Input: part model. Units: mm. Frame: model coordinates. A direction names the side the tool comes from. Round coordinates to 2 decimals unless told otherwise and drop trailing zeros. Loops run counter-clockwise (first coordinate to the right, second up) from the corner with the lowest first, then second, coordinate; pieces in that order, holes last. Notation, with made-up numbers: (59.25, 42) -> (78.25, 42) arc R17 ccw to (78.25, 67) -> close; hole circle Ø9 at (-30.5, -14). An arc over 180 degrees is marked (long way). Answer as a JSON object with one key per item and string values. Group by question number.
Item 1: Draft query along Y for faces 5 (the flat face through (-8, 27, 3.175)), 6 (the cylindrical face through (-51.7, 122.3, 0)), 7 (the cylindrical face through (45.26, 111.96, 0.83)), 8 (the cylindrical face through (40.365, 31.913, 0.827)). Return one class per face: released by +Y, released by -Y, zero draft, split by the parting line, or undercut.
Item 2: Section query C-C on y = 71. Return loops of the section in (x, z) (3 decimals).
Item 3: Pin query (flat end, axial travel): pin 1 (6 mm diameter, centred on x = 42.52, y = 30.54, fed in from +Z) (3 decimals); pin 2 (8 mm diameter, centred on x = -96.27, y = 37.1, fed in from -Z); pin 3 (4 mm diameter, centred on x = 46.02, y = 109.52, fed in from +Z); pin 4 (2 mm diameter, centred on x = 34, z = 0, fed in from +Y). Return the tip coordinate at first contact, or that it passes through.
Item 4: Section query A-A on x = 25.5. Return loops of the section in (y, z) (3 decimals), and give its area (3 significant figures).
Item 5: Set-up query: faces 1 (the flat face through (-8, 27, -3.175)), 2 (the cylindrical face through (-8.13, 123.04, -2.37)), 3 (the flat face through (-37.823, -58.096, 0.044)), 4 (the cylindrical face through (-48.07, -24.55, -0.04)). Return all of +Z, -Z, +X, -X, +Y, -Y with unobstructed straight access to the full face (end or side cutting, diameter ignored); none if empty.
Item 6: Section query B-B on z = 1.25. Count the separate pieces of the cut face and the enclosed holes in it, and give its area (3 significant figures).
Item 7: Material intervals for line 1 (Y direction, x = -13, z = -1.25); line 2 (Y direction, x = -41, z = 0.5); line 3 (X direction, y = 78.5, z = 0.5), sorted ascending. Write a range as [from, to].
Autodesk Inventor part; units mm, degrees
ref_plane "YZ Plane" through (0, 0, 0) normal (1, 0, 0) x (0, 1, 0)
ref_plane "XZ Plane" through (0, 0, 0) normal (0, 1, 0) x (-1, 0, 0)
ref_plane "XY Plane" through (0, 0, 0) normal (0, 0, 1) x (1, 0, 0)
sketch "Sketch1" plane through (0, 0, 0) normal (0, 0, 1) x (1, 0, 0)
  line L0 (-176.0344, 0) -> (115.3938, 0)
  line L1 (0, -134.9094) -> (0, 212.5709)
  line L2 (0, 0) -> (-134.4018, 134.4018) construction
  circle A0 centre (0, 0) radius 16.51
  circle A1 centre (-64.8398, 5.6727) radius 6.35 construction
  circle A2 centre (46.0238, 46.0238) radius 6.35 construction
  arc A3 (-51.2387, -16.9675) -> (-59.3872, -5.1957) centre (-75.3511, -24.9522) ccw
  arc A4 (48.833, 34.1932) -> (50.1576, 19.9378) centre (73.7612, 29.3203) ccw
  circle A5 centre (0, 0) radius 53.975 construction
  circle A6 centre (-50.2894, 50.2894) radius 14.2875
  circle A7 centre (-26.9875, 87.3943) radius 11.1125
  circle A8 centre (13.589, 89.6653) radius 14.2875
  arc A9 (51.2312, 117.4993) -> (-105.7834, 37.5874) centre (-4.3145, 32.4274) ccw
  line L3 (-103.0059, 30.3685) -> (-71.575, -1.0624)
  line L4 (55.5488, 46.0238) -> (55.5488, 109.5238)
  arc A10 (55.5488, 109.5238) -> (51.2312, 117.4993) centre (46.0238, 109.5238) ccw
  arc A11 (-105.7834, 37.5874) -> (-103.0059, 30.3685) centre (-96.2707, 37.1036) ccw
  arc A12 (-71.575, -1.0624) -> (-63.9628, -3.8118) centre (-64.8398, 5.6727) ccw
  arc A13 (51.4486, 38.1945) -> (55.5488, 46.0238) centre (46.0238, 46.0238) ccw
  line L5 (0, 0) -> (-64.8398, 5.6727) construction
  arc A14 (-59.3872, -5.1957) -> (-63.9628, -3.8118) centre (-63.3782, -10.1348) ccw
  arc A15 (51.4486, 38.1945) -> (48.833, 34.1932) centre (55.0651, 32.975) ccw
  line L6 (0, 0) -> (46.0238, 46.0238) construction
  line L7 (-59.3872, -5.1957) -> (0, 0) construction
  line L8 (48.833, 34.1932) -> (0, 0) construction
  line L9 (0, 0) -> (-28.2338, -77.5716) construction
  line L10 (0.6691, -79.3887) -> (9.0934, -56.243)
  line L11 (-43.1182, -37.2395) -> (-51.5426, -60.3852)
  arc A16 (-51.2387, -16.9675) -> (-43.9184, -31.3763) centre (0, 0) ccw
  arc A17 (13.4752, -52.2659) -> (50.1576, 19.9378) centre (0, 0) ccw
  arc A18 (-48.7265, -68.0701) -> (-6.4279, -83.4655) centre (17.2205, 47.3129) ccw
  arc A19 (-43.1182, -37.2395) -> (-43.9184, -31.3763) centre (-49.0853, -35.0676) ccw
  arc A20 (-51.5426, -60.3852) -> (-48.7265, -68.0701) centre (-45.5755, -62.557) ccw
  arc A21 (-6.4279, -83.4655) -> (0.6691, -79.3887) centre (-5.298, -77.2168) ccw
  arc A22 (13.4752, -52.2659) -> (9.0934, -56.243) centre (15.0605, -58.4148) ccw
  circle A23 centre (-17.0625, 17.0625) radius 4.7625 construction
  point P0 (55.5488, 114.5184)
  point P1 (-105.911, 33.2736)
  point P2 (-1.1237, -84.3143)
  point P3 (-41.9333, -33.9838)
  point P4 (-53.3354, -65.3108)
  point P5 (10.2784, -52.9873)
  dimension "d1" = 33.02
  dimension "d5" = 12.7
  dimension "d11" = 25.4
  dimension "d14" = 45
  dimension "d16" = 107.95
  dimension "d19" = 28.575
  dimension "d22" = 22.225
  dimension "d25" = 43.815
  dimension "d27" = 28.575
  dimension "d29" = 40.64
  dimension "d30" = 9.525
  dimension "d31" = 9.525
  dimension "d34" = 63.5
  dimension "d35" = 101.6
  dimension "d36" = 44.45
  dimension "d38" = 6.35
  dimension "d39" = 6.35
  dimension "d43" = 65.0875
  dimension "d44" = 130
  dimension "d45" = 5
  dimension "d46" = 35
  dimension "d57" = 20
  dimension "d58" = 27.7812
  dimension "d60" = 33.3375
  dimension "d61" = 33.3375
  dimension "d63" = 82.55
  dimension "d64" = 6.35
  dimension "d83" = 24.13
  dimension "d84" = 9.525
  dimension "d85" = 46.99
  dimension "d86" = 26.9875
  dimension "d87" = 13.589
extrude "Base" add sketch "Sketch1" along normal mid plane 6.35 contours L3 A11 A9 L1 A8 A0 L0 | L0 A0 L1 A21 A18 A20 L11 A19 A16 A3 A14 A12 L3 | L1 A8 A9 A10 L4 A13 A15 A4 A17 L0 A0 | A0 L0 A17 A22 L10 A21 L1
sketch "Sketch2" plane through (0, 0, -3.175) normal (0, 0, -1) x (-1, 0, 0)
  arc A0 (103.0059, 30.3685) -> (105.7834, 37.5874) centre (96.2707, 37.1036) ccw
  arc A1 (-51.2312, 117.4993) -> (-55.5488, 109.5238) centre (-46.0238, 109.5238) ccw
  arc A2 (-50.1576, 19.9378) -> (-13.4752, -52.2659) centre (0, 0) ccw
  line L0 (141.1514, 0) -> (-101.0644, 0)
  line L1 (0, -127.0857) -> (0, 177.5463)
  line L2 (0, 0) -> (11.1042, 126.9216) construction
  line L3 (0, 0) -> (77.2258, 92.0341) construction
  dimension "d88" = 5
  dimension "d89" = 40
  dimension "d90" = 127.4064
  dimension "d91" = 120.142
hole "Standoff Holes" at (46.0238, 109.5238, -3.175) at (-96.2707, 37.1036, -3.175) at (-77.2258, 92.0341, -3.175) at (-11.1042, 126.9216, -3.175) direction (0, 0, 1) diameter 5.1054 end through all counterbore diameter 9.779 counterbore depth 1.5875
sketch "Sketch4" plane through (0, 0, 3.175) normal (0, 0, 1) x (1, 0, 0)
  line L0 (9.0934, -56.243) -> (0.6691, -79.3887)
  arc A0 (-46.8486, -63.1399) -> (-40.4997, -65.4507) centre (-43.6742, -64.2953) ccw
  arc A1 (-11.0463, -76.1709) -> (-4.6974, -78.4817) centre (-7.8719, -77.3263) ccw
  arc A2 (-35.0701, -50.5331) -> (-41.4191, -48.2223) centre (-38.2446, -49.3777) ccw
  arc A3 (0.7322, -63.5641) -> (-5.6168, -61.2532) centre (-2.4423, -62.4087) ccw
  line L1 (-40.4997, -65.4507) -> (-35.0701, -50.5331)
  line L2 (-46.8486, -63.1399) -> (-41.4191, -48.2223)
  line L3 (-11.0463, -76.1709) -> (-5.6168, -61.2532)
  line L4 (0.7322, -63.5641) -> (-4.6974, -78.4817)
  line L5 (-7.8719, -77.3263) -> (-43.6742, -64.2953) construction
  arc A4 (-48.7265, -68.0701) -> (-6.4279, -83.4655) centre (17.2205, 47.3129) ccw
  arc A5 (33.6371, -20.1122) -> (39.9861, -22.423) centre (36.8116, -21.2676) ccw
  arc A6 (45.4156, -7.5054) -> (39.0667, -5.1946) centre (42.2412, -6.35) ccw
  line L6 (39.9861, -22.423) -> (45.4156, -7.5054)
  line L7 (39.0667, -5.1946) -> (33.6371, -20.1122)
  line L8 (-140.2473, 0) -> (100.9137, 0)
  line L9 (0, -129.1287) -> (0, 177.8868)
  arc A7 (13.4752, -52.2659) -> (50.1576, 19.9378) centre (0, 0) ccw
  dimension "d66" = 6.7564
  dimension "d70" = 15.875
  dimension "d71" = 38.1
  dimension "d72" = 5.353
  dimension "d73" = 2.3813
  dimension "d74" = 15.875
  dimension "d75" = 6.7564
  dimension "d76" = 15.875
  dimension "d77" = 6.35
  dimension "d78" = 45.2437
extrude "Tensioning Slots" cut sketch "Sketch4" against normal through all
sketch "Sketch5" plane through (0, 0, 3.175) normal (0, 0, 1) x (1, 0, 0)
  circle A0 centre (0, 0) radius 16.51
  circle A1 centre (-50.2894, 50.2894) radius 14.2875
  arc A2 (13.4752, -52.2659) -> (50.1576, 19.9378) centre (0, 0) ccw
  line L0 (-71.575, -1.0624) -> (-103.0059, 30.3685)
  line L1 (0, 0) -> (-50.2894, 50.2894) construction
  circle A3 centre (-17.0625, 17.0625) radius 4.7625
  line L2 (-140.2473, 0) -> (100.9137, 0)
  line L3 (0, -127.0857) -> (0, 177.5463)
  dimension "d79" = 9.525
  dimension "d80" = 24.13
extrude "Idler Bearing Hole" cut sketch "Sketch5" against normal through all contours A3
sketch "Sketch6" plane through (0, 0, -3.175) normal (0, 0, -1) x (-1, 0, 0)
  arc A0 (63.9628, -3.8118) -> (71.575, -1.0624) centre (64.8398, 5.6727) ccw
  arc A1 (-55.5488, 46.0238) -> (-51.4486, 38.1945) centre (-46.0238, 46.0238) ccw
  line L0 (140.2473, 0) -> (-100.9137, 0)
  line L1 (0, -127.0857) -> (0, 177.5463)
  circle A2 centre (-42.5172, 30.5409) radius 6.35 construction
  circle A3 centre (52.2014, -3.9338) radius 6.35 construction
  arc A4 (-50.1576, 19.9378) -> (-13.4752, -52.2659) centre (0, 0) ccw
  line L2 (0, 0) -> (-42.5172, 30.5409) construction
  line L3 (0, 0) -> (52.2014, -3.9338) construction
  dimension "d92" = 12.7
  dimension "d93" = 15.875
  dimension "d94" = 15.875
  dimension "d102" = 52.3494
  dimension "d103" = 52.3494
hole "Standoff holes to motor plate" at (42.5172, 30.5409, -3.175) at (-52.2014, -3.9338, -3.175) direction (0, 0, 1) diameter 5.1054 end through all counterbore diameter 9.779 counterbore depth 1.5875
properties part number "front plate"
Solved:
{
 "1": {"face 5": "zero draft", "face 6": "released by +Y", "face 7": "undercut", "face 8": "undercut"},
 "2": {"outline": "(-98.308, -3.175) -> (55.549, -3.175) -> (55.549, 3.175) -> (-98.308, 3.175) -> close"},
 "3": {"pin 1": "z = 3.175", "pin 2": "z = -1.59", "pin 3": "through", "pin 4": "y = 126.93"},
 "4": {"outline": "(-47.572, -3.175) -> (81.775, -3.175) -> (81.775, 3.175) -> (-47.572, 3.175) -> close; (97.556, -3.175) -> (129.554, -3.175) -> (129.554, 3.175) -> (97.556, 3.175) -> close", "area": "1,020 mm²"},
 "5": {"face 1": "-Z, +X, -X, +Y, -Y", "face 2": "-Z", "face 3": "+Z, -Z", "face 4": "+Z, -Z, -X"},
 "6": {"separate pieces": "1", "enclosed holes": "14", "area": "21,500 mm²"},
 "7": {"line 1": "[-82.1, -10.18], [10.18, 14.58], [19.55, 125.21], [128.63, 133.66]", "line 2": "[-72.16, -66.36], [-47.42, 39.43], [61.14, 127.17]", "line 3": "[-94.87, -33.65], [-20.33, 4.67], [22.5, 55.55]"}
}
